Input: dimensioned drawing with shaded views. Units: mm. Origin: part minimum x, y, z. A direction names the side the tool comes from. Round coordinates to 2 decimals unless told otherwise and drop trailing zeros. Order: outer loops, then holes, each group sorted by start corner. A loop starts at its lowest first (then second) coordinate and runs counter-clockwise, first axis right, second up. Notation, with made-up numbers: M 80,28 L 97,28 A24 cw 97,49 Z; hole C -16.75,-1.75 d6. An arc over 180 degrees is marked long. Use one line per item in the form item = value. Start each with the question number.
Q1. Pull-direction query (Y, two-part tool) for the marked faces 1, 2 and 3; classes: pulls with the +Y half, pulls with the -Y half, needs draft (parallel to the pull), parting line crosses it, or undercut.
Q2. Section B-B (x = 12). Return the cut outline in (y, z), plus the area to 3 significant figures.
Q3. Contact query for flat-ended pins moving along their axis: pin 1 (10 mm diameter, centred on y = 42, z = 14.5, fed in from -X) (1 decimal); pin 2 (6 mm diameter, centred on x = 45, y = 6, fed in from +Z); pin 3 (3 mm diameter, centred on x = 29.5, z = 19, fed in from +Y). Output: stop coordinate, or through.
Q4. Reachability of the marked faces 4, 5 and 6 from +Z, -Z, +X, -X, +Y, -Y: full face, straight path, thin tool, end or side. Return the list, or none.
Q5. Material intervals for probe 1 along Y at (x, z) = (30, 23.25); probe 2 along Y at (x, z) = (28.5, 14.25); probe 3 along Y at (x, z) = (4, 11.5), sorted ascending.
Q6. Section C-C (z = 7.25). Give the number of separate pieces and of enclosed holes in the cut face.
Q7. Section D-D (y = 44). Return the cut outline in (x, z) (1 decimal).
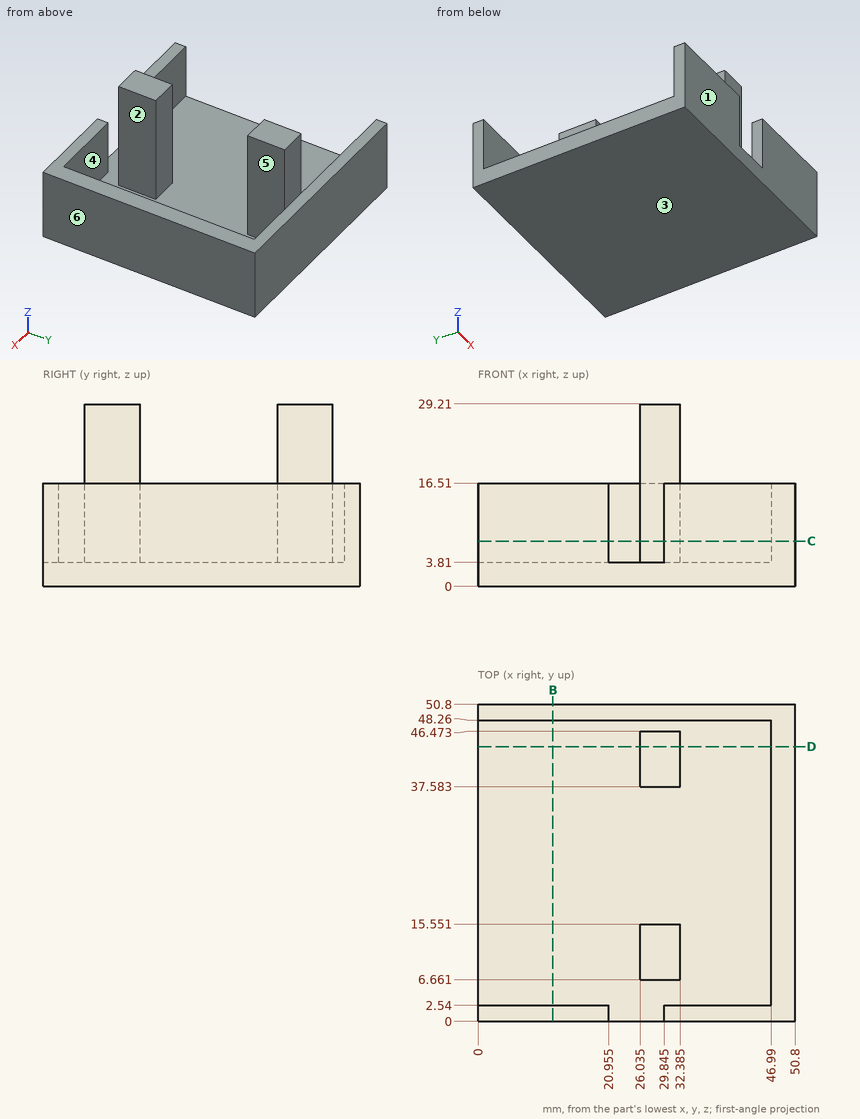
Results list:
q1.face_1 = pulls with the -Y half
q1.face_2 = undercut
q1.face_3 = needs draft
q2.outline = M 0,0 L 50.8,0 L 50.8,16.51 L 48.26,16.51 L 48.26,3.81 L 2.54,3.81 L 2.54,16.51 L 0,16.51 Z
q2.area = 258 mm2
q3.pin_1 = 26
q3.pin_2 = 16.51
q3.pin_3 = 46.47
q4.face_4 = +Z, -X
q4.face_5 = +Z
q4.face_6 = +Z, -Z, +X, +Y, -Y
q5.probe_1 = 6.66 to 15.55, 37.58 to 46.47
q5.probe_2 = 6.66 to 15.55, 37.58 to 46.47, 48.26 to 50.8
q5.probe_3 = 0 to 2.54, 48.26 to 50.8
q6.separate_pieces = 4
q6.enclosed_holes = 0
q7.outline = M 0,0 L 50.8,0 L 50.8,16.5 L 47,16.5 L 47,3.8 L 32.4,3.8 L 32.4,29.2 L 26,29.2 L 26,3.8 L 0,3.8 Z
